Here's how the part is built. I have some questions about the finished solid (model axes, mm). Give positions to 0.01 mm unless a question says otherwise; leave off trailing zeros. Write each loop counter-clockwise with the first axis right and the second up, starting at its lowest first coordinate (ties: lowest second). Pieces come first, ordered by that corner, then holes. Notation, with made-up numbers: (36, 0) -> (65, 0) arc R33 ccw to (65, 28) -> close; hole circle Ø7 at (-3, -31). An arc over 180 degrees is marked (long way). Use CSV: the item, a comma, the result in double quotes. Start each with the question number.
(1) I need wall thicknesses on L1, parallel to X at y = 11, z = 0.25; L2, parallel to Y at x = -47.51, z = 1.2; L3, parallel to Y at x = -46.5, z = 0.25. Which ranges of each line are inside material? Lowest first, please. Write a range as [from, to].
(2) Suppose I cut it at A-A on x = 0. List the corners of the cut face in (y, z) for me (3 decimals).
(3) For pin 1 Ø4 at (x, y) = (47.51, -11.26) entering from -Z, with a flat end and sliding along its axis, tell me the tip position at first contact or that it passes through.
(4) Suppose I cut it at B-B on y = -2.35. List the corners of the cut face in (x, z) for me (3 decimals).
(5) Suppose I cut it at C-C on z = 0.5. Give the number of separate pieces and of enclosed holes in the cut face, plus the area to 3 significant figures.
from build123d import *

# Parameters (mm, degrees)
SKETCH_W        = 103
SKETCH_H        = 30.3
PAD_DEPTH       = 1.62
SKETCH001_R     = 2.1
POCKET_DEPTH    = 5
SKETCH002_R     = 3.675
POCKET001_DEPTH = 5
FILLET_R        = 4


with BuildPart() as part:
    # Sketch → Pad (new body)
    with BuildSketch(Plane.XY):
        Rectangle(SKETCH_W, SKETCH_H)
    extrude(amount=PAD_DEPTH)

    # Sketch001 → Pocket (cut)
    with BuildSketch(Plane.XY.offset(1.62)):
        with Locations((-47.51, 11.26)):
            Circle(SKETCH001_R)
        with Locations((47.51, 11.26)):
            Circle(SKETCH001_R)
        with Locations((-47.51, -11.26)):
            Circle(SKETCH001_R)
        with Locations((47.51, -11.26)):
            Circle(SKETCH001_R)
    extrude(amount=-POCKET_DEPTH, mode=Mode.SUBTRACT)

    # Sketch002 → Pocket001 (cut)
    with BuildSketch(Plane.XY.offset(1.62)):
        with Locations((-32.004, -2.35)):
            Circle(SKETCH002_R)
        with Locations((-16.002, -2.35)):
            Circle(SKETCH002_R)
        with Locations((0, -2.35)):
            Circle(SKETCH002_R)
        with Locations((16.002, -2.35)):
            Circle(SKETCH002_R)
        with Locations((32.004, -2.35)):
            Circle(SKETCH002_R)
    extrude(amount=-POCKET001_DEPTH, mode=Mode.SUBTRACT)

    # Fillet
    fillet_edges = [part.edges().sort_by_distance(p)[0] for p in [
        (-51.5, -15.15, 0.81),
        (-51.5, 15.15, 0.81),
        (51.5, -15.15, 0.81),
        (51.5, 15.15, 0.81),
    ]]
    fillet(fillet_edges, radius=FILLET_R)


solid = part.part
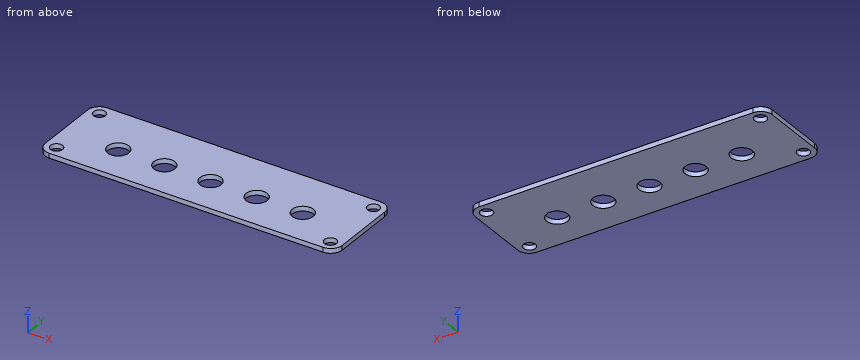
Geometry says:
1,L1,"[-51.5, -49.59], [-45.43, 45.43], [49.59, 51.5]"
1,L2,"[-15.15, -13.36], [-9.16, 9.16], [13.36, 15.15]"
1,L3,"[-15.15, -13.1], [-9.42, 9.42], [13.1, 15.15]"
2,outline,"(-15.15, 0) -> (-6.025, 0) -> (-6.025, 1.62) -> (-15.15, 1.62) -> close; (1.325, 0) -> (15.15, 0) -> (15.15, 1.62) -> (1.325, 1.62) -> close"
3,pin 1,"through"
4,outline,"(-51.5, 0) -> (-35.679, 0) -> (-35.679, 1.62) -> (-51.5, 1.62) -> close; (-28.329, 0) -> (-19.677, 0) -> (-19.677, 1.62) -> (-28.329, 1.62) -> close; (-12.327, 0) -> (-3.675, 0) -> (-3.675, 1.62) -> (-12.327, 1.62) -> close; (3.675, 0) -> (12.327, 0) -> (12.327, 1.62) -> (3.675, 1.62) -> close; (19.677, 0) -> (28.329, 0) -> (28.329, 1.62) -> (19.677, 1.62) -> close; (35.679, 0) -> (51.5, 0) -> (51.5, 1.62) -> (35.679, 1.62) -> close"
5,separate pieces,"1"
5,enclosed holes,"9"
5,area,"2,840 mm²"
